Autodesk Inventor part; units mm, degrees
ref_plane "YZ Plane" through (0, 0, 0) normal (1, 0, 0) x (0, 1, 0)
ref_plane "XZ Plane" through (0, 0, 0) normal (0, 1, 0) x (-1, 0, 0)
ref_plane "XY Plane" through (0, 0, 0) normal (0, 0, 1) x (1, 0, 0)
ref_plane "Arbeitsebene1" through (-28.1717, -118.9029, 44.8795) normal (0, -1, 0) x (1, 0, 0)
sketch "Skizze1" plane through (-28.1717, -118.9029, 44.8795) normal (0, -1, 0) x (1, 0, 0)
  line L0 (-16.24, -39.62) -> (-16.8, -39.62)
  arc A0 (-16.24, -39.62) -> (-14.94, -38.32) centre (-16.24, -38.32) ccw
  line L1 (-14.94, -38.32) -> (-14.94, -31.98)
  arc A1 (-14.94, -31.98) -> (-16.24, -30.68) centre (-16.24, -31.98) ccw
  line L2 (-16.24, -30.68) -> (-16.8, -30.68)
  arc A2 (-16.8, -30.68) -> (-18.1, -31.98) centre (-16.8, -31.98) ccw
  line L3 (-18.1, -38.32) -> (-18.1, -31.98)
  arc A3 (-18.1, -38.32) -> (-16.8, -39.62) centre (-16.8, -38.32) ccw
  arc A4 (-16.8, -30.98) -> (-17.8, -31.98) centre (-16.8, -31.98) ccw
  line L4 (-16.24, -30.98) -> (-16.8, -30.98)
  arc A5 (-15.24, -31.98) -> (-16.24, -30.98) centre (-16.24, -31.98) ccw
  line L5 (-15.24, -31.98) -> (-15.24, -38.32)
  arc A6 (-16.24, -39.32) -> (-15.24, -38.32) centre (-16.24, -38.32) ccw
  line L6 (-16.8, -39.32) -> (-16.24, -39.32)
  arc A7 (-17.8, -38.32) -> (-16.8, -39.32) centre (-16.8, -38.32) ccw
  line L7 (-17.8, -38.32) -> (-17.8, -31.98)
  point P0 (28.1717, -44.8795)
extrude "Extrusion1" add sketch "Skizze1" against normal blind 10
equation "\"d_tol\" = 0.3"
equation "\"d_wand\" = 1.5"
equation "\"r_rasp_pi\" = 3"
equation "\"D_oct\" = 3621.32034"
equation "\"d_traeger\" = 625"
equation "\"l_rasp_pi\" = 85"
equation "\"w_kamera_vert\" = 41deg"
equation "\"w_kamera_hori\" = 66deg"
equation "\"D_hexadeca\" = 7541.00924"
equation "\"b_rasp_pi\" = 56"
properties part number "Camera_Assembly_Electrical"
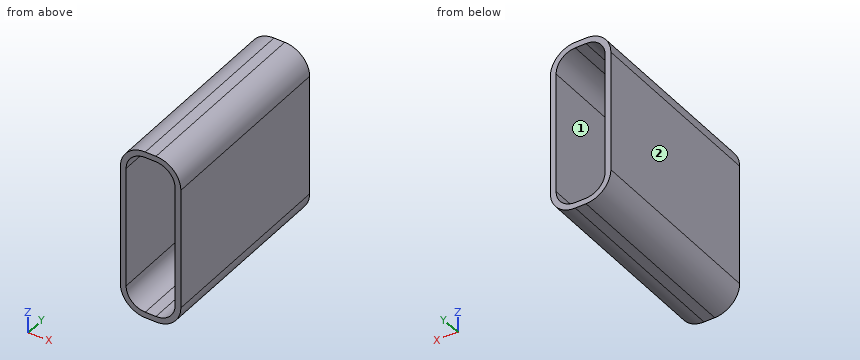
Here's how the part is built. I have some questions about the finished solid (model axes, mm). Face numbers are marked on the shaded views. A direction names the side the tool comes from. Round coordinates to 2 decimals unless told otherwise and drop trailing zeros. Order: outer loops, then holes, each group sorted by start corner. A loop starts at its lowest first (then second) coordinate and runs counter-clockwise, first axis right, second up. Notation, with made-up numbers: M 35,79.25 L 73,79.25 A21 ccw 73,105.25 Z; hole C 65,2 d8. An arc over 180 degrees is marked long. Use CSV: the item, a comma, the result in double quotes.
1) I want a section at A-A (x = -45.7). List the corners of the cut face in (y, z) for me.
Taken from the geometry:
outline,"M -118.9,5.48 L -108.9,5.48 L -108.9,5.87 L -118.9,5.87 Z; M -118.9,13.58 L -108.9,13.58 L -108.9,13.98 L -118.9,13.98 Z"
2) I'm going to push a flat-ended pin straight in: P1, Ø1.5, axis at x = -43.5, z = 6.5, coming from the -Y side. Where does the tip first touch, or does it pass through?
Taken from the geometry:
P1,"y = -118.9"
3) I want a section at B-B (y = -117). List the corners of the cut face in (x, z) for me.
Taken from the geometry:
outline,"M -46.27,6.56 A1.3 ccw -44.97,5.26 L -44.41,5.26 A1.3 ccw -43.11,6.56 L -43.11,12.9 A1.3 ccw -44.41,14.2 L -44.97,14.2 A1.3 ccw -46.27,12.9 Z; hole M -45.97,6.56 A1 ccw -44.97,5.56 L -44.41,5.56 A1 ccw -43.41,6.56 L -43.41,12.9 A1 ccw -44.41,13.9 L -44.97,13.9 A1 ccw -45.97,12.9 Z"
4) I need wall thicknesses on line 1 along Z through (x, y) = (-44.8, -114.5); line 2 along X through (y, z) = (-115.25, 10.25); line 3 along Z through (x, y) = (-45.6, -113.75). Which ranges of each line are inside material? Lowest first, please. Write a range as [from, to].
Taken from the geometry:
line 1,"[5.26, 5.56], [13.9, 14.2]"
line 2,"[-46.27, -45.97], [-43.41, -43.11]"
line 3,"[5.42, 5.78], [13.68, 14.04]"
5) I want a section at C-C (z = 10.75). List the corners of the cut face in (x, y) for me.
Taken from the geometry:
outline,"M -46.27,-118.9 L -45.97,-118.9 L -45.97,-108.9 L -46.27,-108.9 Z; M -43.41,-118.9 L -43.11,-118.9 L -43.11,-108.9 L -43.41,-108.9 Z"
6) On a 3-axis mill with a long thin cutter (end or side, diameter ignored), from which of +Z, -Z, +X, -X, +Y, -Y can I reach the whole of each face in a straight line? I mean the marked faces 1 and 2. Say none if no direction works.
Taken from the geometry:
face 1,"+Y, -Y"
face 2,"+Z, -Z, -X, +Y, -Y"
